For this review, take the finished solid that the model builds, in its own axes (mm). A direction names the side the tool comes from. Coordinates: 2 decimals unless noted, no trailing zeros. Loops run counter-clockwise (first coordinate to the right, second up) from the corner with the lowest first, then second, coordinate; pieces in that order, holes last. Notation, with made-up numbers: M -20,-33.5 L -12,-33.5 A12 cw -12,-15.5 Z; hole C 64.25,79.25 d7. An arc over 180 degrees is marked long. Answer as a JSON object with one key per item and string values. Group by question number.
Item 1: Insertion check: pin 1 (0.9 mm diameter, centred on y = -50.5, z = 2, fed in from +X); pin 2 (0.9 mm diameter, centred on y = -51, z = 1.5, fed in from -X); pin 3 (1.2 mm diameter, centred on x = -9.5, z = 1.5, fed in from -Y). Each pin has a flat end and moves straight along its axis. Give the tip position at first contact, or say it passes through.
Item 2: Mouldability with a two-part tool opening along X and no side actions: class faces 1 (the face through (52.094, 26.454, 1.521)), 2 (the face through (-21.705, 5.786, 1.479)), 3 (the face through (-16, -52.5, 1)) as +X half, -X half, draft (parallel to the pull), parting line (faces both ways), or undercut.
Item 3: Add section C-C (y = -9.5). State the section outline as (x, z) points, then the cut area to 3 significant figures.
Item 4: Add section D-D (x = 20). State the section outline as (y, z) points.
Item 5: Add section B-B (z = 2.2). Count the separate pieces of the cut face and the enclosed holes in it, then the cut area to 3 significant figures.
Item 6: Tool access review of faces 4 (the face through (-21.347, -44.715, 1.521)), 5 (the face through (48.23, 20.11, 1.52)), 6 (the face through (-10.78, -44.43, 1.52)), 7 (the face through (-5.704, -1.503, 1.479)): name each direction out of +Z, -Z, +X, -X, +Y, -Y from which nothing blocks a thin tool from reaching the whole face with its end or side.
Item 7: Add section A-A (y = -42.5). State the section outline as (x, z) points.
Item 8: Wall thickness on L1, parallel to X at y = -7, z = 2.7; L2, parallel to Y at x = -17, z = 1.6; L3, parallel to X at y = 5, z = 2.15: over which ranges is each line inside the solid? List them lowest first. Write a range as from..to.
from build123d import *

# Parameters (mm, degrees)
SKETCH_1_R          = 1.5
EXTRUDE_1_DEPTH     = 3
FILLET_1_R          = 2
FILLET_2_R          = 1.5
EXTRUDE_2_DEPTH     = 3
CUT_EXTRUDE_2_DEPTH = 10
EXTRUDE_3_DEPTH     = 3
FILLET_4_R          = 1.5
SKETCH_8_R          = 1.5
CUT_EXTRUDE_3_DEPTH = 3
SKETCH_9_R          = 1
CUT_EXTRUDE_4_DEPTH = 10
SKETCH_10_R         = 1.5
CUT_EXTRUDE_5_DEPTH = 10
SKETCH_11_R         = 1.5
CUT_EXTRUDE_6_DEPTH = 75.756148202


with BuildPart() as part:
    # 草图1 → 凸台-拉伸1 (new body)
    with BuildSketch(Plane.XY):
        with BuildLine():
            ThreePointArc((-0.817087424, -2.886584165), (2.886584165, -0.817087424), (0.817087424, 2.886584165))
            Line((0.817087424, 2.886584165), (-1.760091504, 3.616090173))
            Line((-1.760091504, 3.616090173), (64.410402882, 27.700180516))
            Line((64.410402882, 27.700180516), (62.358282022, 33.338336241))
            Line((62.358282022, 33.338336241), (-11.628300128, 6.409422603))
            Line((-11.628300128, 6.409422603), (-19.389001732, 8.606196131))
            ThreePointArc((-19.389001732, 8.606196131), (-23.09267332, 6.53669939), (-21.023176579, 2.833027801))
            Line((-21.023176579, 2.833027801), (-19, 2.260339792))
            Line((-19, 2.260339792), (-19, -52.5))
            Line((-19, -52.5), (-13, -52.5))
            Line((-13, -52.5), (-13, 0.561957115))
            Line((-13, 0.561957115), (-0.817087424, -2.886584165))
        make_face()
        with Locations((-20.206089155, 5.719611966)):
            Circle(SKETCH_1_R, mode=Mode.SUBTRACT)
        Circle(SKETCH_1_R, mode=Mode.SUBTRACT)
    extrude(amount=EXTRUDE_1_DEPTH)

    # 圆角1
    fillet_1_edges = [part.edges().sort_by_distance(p)[0] for p in [
        (-11.628300128, 6.409422603, 1.5),
        (-13, 0.561957115, 1.5),
        (-19, 2.260339792, 1.5),
    ]]
    fillet(fillet_1_edges, radius=FILLET_1_R)

    # 圆角2
    fillet_2_edges = [part.edges().sort_by_distance(p)[0] for p in [
        (-1.760091504, 3.616090173, 1.5),
    ]]
    fillet(fillet_2_edges, radius=FILLET_2_R)

    # 草图3 → 凸台-拉伸2 (add)
    with BuildSketch(Plane.XY.offset(3)):
        with BuildLine():
            Line((-21, -49.5), (-23.5, -49.5))
            Line((-23.5, -49.5), (-19, -39.5))
            Line((-19, -39.5), (-19, -49.5))
            ThreePointArc((-19, -49.5), (-20, -48.5), (-21, -49.5))
        make_face()
        with BuildLine():
            Line((-13, -49.5), (-13, -39.5))
            Line((-13, -39.5), (-8.5, -49.5))
            Line((-8.5, -49.5), (-11, -49.5))
            ThreePointArc((-11, -49.5), (-12, -48.5), (-13, -49.5))
        make_face()
    extrude(amount=-EXTRUDE_2_DEPTH)

    # 草图7 → 切除-拉伸2 (cut)
    with BuildSketch(Plane.XY.offset(3)):
        Polygon((53.134091432, 23.595938796), (64.410402882, 27.700180516), (62.358282022, 33.338336241), (51.081970572, 29.234094521), align=None)
    extrude(amount=-CUT_EXTRUDE_2_DEPTH, mode=Mode.SUBTRACT)

    # 草图4 → 凸台-拉伸3 (add)
    with BuildSketch(Plane.XY.offset(3)):
        Polygon((42.624736985, 26.155913231), (47.23683228, 31.027111953), (48.26289271, 28.208034091), (51.081970572, 29.234094521), (53.134091432, 23.595938796), (50.31501357, 22.569878366), (51.341074, 19.750800504), (44.676857845, 20.517757506), align=None)
    extrude(amount=-EXTRUDE_3_DEPTH)

    # 圆角4
    fillet_4_edges = [part.edges().sort_by_distance(p)[0] for p in [
        (44.676857845, 20.517757506, 1.5),
        (42.624736985, 26.155913231, 1.5),
        (-19, -39.5, 1.5),
    ]]
    fillet(fillet_4_edges, radius=FILLET_4_R)

    # 草图8 → 切除-拉伸3 (cut)
    with BuildSketch(Plane.XY.offset(3)):
        with Locations((42.711104794, 22.994815225)):
            Circle(SKETCH_8_R)
    extrude(amount=-CUT_EXTRUDE_3_DEPTH, mode=Mode.SUBTRACT)

    # 草图9 → 切除-拉伸4 (cut)
    with BuildSketch(Plane.XY.offset(3)):
        with Locations((47.920872567, 29.147726712)):
            Circle(SKETCH_9_R)
        with Locations((50.657033713, 21.630185745)):
            Circle(SKETCH_9_R)
    extrude(amount=-CUT_EXTRUDE_4_DEPTH, mode=Mode.SUBTRACT)

    # 草图10 → 切除-拉伸5 (cut)
    with BuildSketch(Plane.XY.offset(3)):
        with Locations((-16, -42.5)):
            Circle(SKETCH_10_R)
    extrude(amount=-CUT_EXTRUDE_5_DEPTH, mode=Mode.SUBTRACT)

    # 草图11 → 切除-拉伸6 (cut, through all)
    with BuildSketch(Plane.XY.offset(3)):
        with Locations((16.399711412, 13.418251212)):
            Circle(SKETCH_11_R)
        with Locations((7.002785205, 9.998049779)):
            Circle(SKETCH_11_R)
        with Locations((29.555408103, 18.206533219)):
            Circle(SKETCH_11_R)
    extrude(amount=-CUT_EXTRUDE_6_DEPTH, mode=Mode.SUBTRACT)


solid = part.part
From the geometry:
{
 "1": {"pin 1": "stops at x = -13", "pin 2": "stops at x = -19", "pin 3": "stops at y = -49.5"},
 "2": {"face 1": "+X half", "face 2": "undercut", "face 3": "draft"},
 "3": {"outline": "M -19,0 L -13,0 L -13,3 L -19,3 Z", "area": "18.0 mm²"},
 "4": {"outline": "M 11.54,0 L 17.92,0 L 17.92,3 L 11.54,3 Z"},
 "5": {"separate pieces": "1", "enclosed holes": "7", "area": "866 mm²"},
 "6": {"face 4": "+Z, -Z, -X", "face 5": "+Z, -Z, -Y", "face 6": "+Z, -Z, +X", "face 7": "+Z, -Z"},
 "7": {"outline": "M -20.35,0 L -17.5,0 L -17.5,3 L -20.35,3 Z; M -14.5,0 L -11.65,0 L -11.65,3 L -14.5,3 Z"},
 "8": {"L1": "x = -19..-13", "L2": "y = -52.5..-43.62, -41.38..7.93", "L3": "x = -23.12..-21.52, -18.89..2.05"}
}
